Job drawing, mm, ordinate dimensions from the low corner. One solid piece. Round coordinates to 2 decimals unless told otherwise and drop trailing zeros. Order: outer loops, then holes, each group sorted by start corner. A loop starts at its lowest first (then second) coordinate and runs counter-clockwise, first axis right, second up. Notation, with made-up numbers: (-21, 87.25) -> (27, 87.25) arc R30 ccw to (27, 113.25) -> close; hole circle Ø9 at (59.25, 17.5). An arc over 180 degrees is marked (long way). Answer as a JSON object with one key per item and string values. Group by question number.
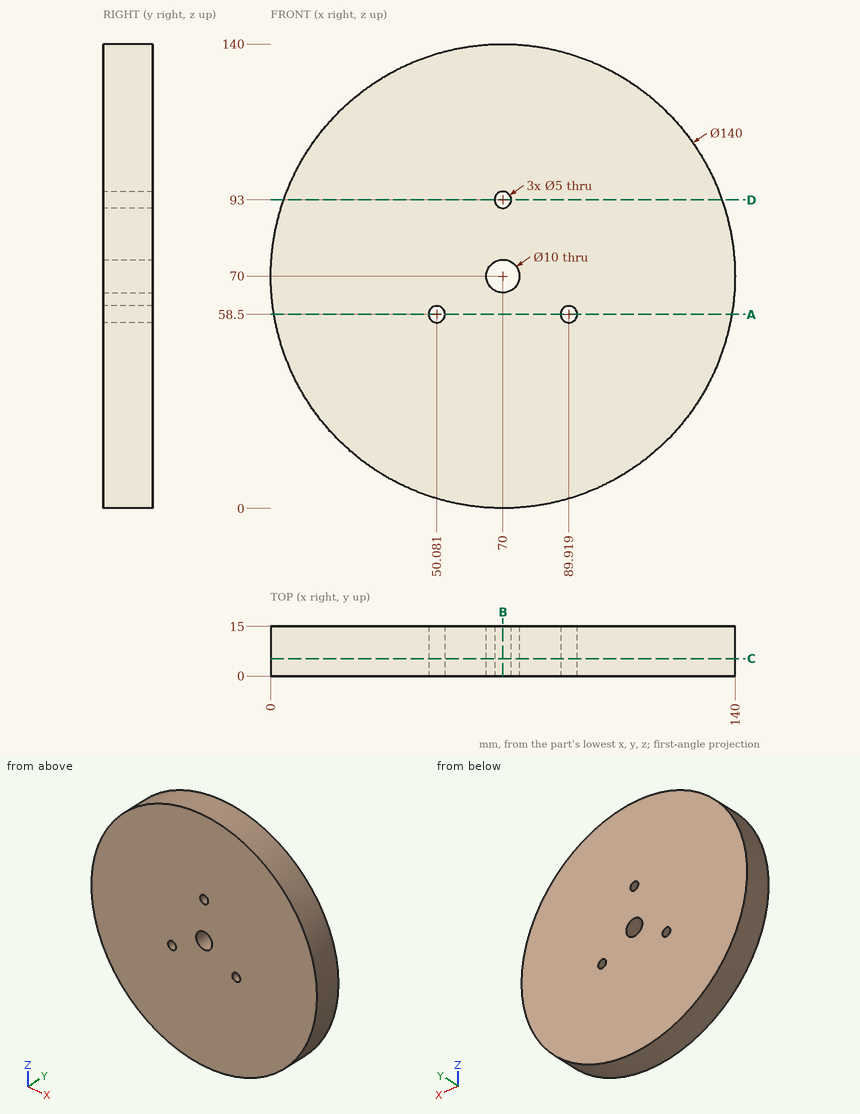
Q1. Band-saw the part on B-B (x = 70). List the corners of the cut face in (y, z), plus the area to 4 significant figures.
Q2. Band-saw the part on A-A (z = 58.5). List the corners of the cut face in (x, y), plus the area to 3 significant figures.
Q3. Band-saw the part on D-D (z = 93). List the corners of the cut face in (x, y), plus the area to 3 significant figures.
Q4. Band-saw the part on C-C (y = 5.25). List the corners of the cut face in (x, z).
Q5. Drop flat-ended pins along their axis: pin 1 Ø6 at (y, z) = (8.5, 33) entering from +X; pin 2 Ø4 at (y, z) = (9, 62) entering from +X; pin 3 Ø4 at (x, y) = (103.5, 1.5) entering from -Z. Give the stop position or say it passes through.
Q6. Wall check: line 1 (Z direction, x = 70, y = 7.75); line 2 (X direction, y = 8, z = 58); line 3 (X direction, y = 4.25, z = 70). Give the ranges that are in metal, low to high. Write a range as [from, to].
Completed:
{
 "1": {"outline": "(0, 0) -> (15, 0) -> (15, 65) -> (0, 65) -> close; (0, 75) -> (15, 75) -> (15, 90.5) -> (0, 90.5) -> close; (0, 95.5) -> (15, 95.5) -> (15, 140) -> (0, 140) -> close", "area": "1,875 mm2"},
 "2": {"outline": "(0.95, 0) -> (47.58, 0) -> (47.58, 15) -> (0.95, 15) -> close; (52.58, 0) -> (87.42, 0) -> (87.42, 15) -> (52.58, 15) -> close; (92.42, 0) -> (139.05, 0) -> (139.05, 15) -> (92.42, 15) -> close", "area": "1,920 mm2"},
 "3": {"outline": "(3.89, 0) -> (67.5, 0) -> (67.5, 15) -> (3.89, 15) -> close; (72.5, 0) -> (136.11, 0) -> (136.11, 15) -> (72.5, 15) -> close", "area": "1,910 mm2"},
 "4": {"outline": "circle Ø140 at (70, 70); hole circle Ø5 at (50.08, 58.5); hole circle Ø10 at (70, 70); hole circle Ø5 at (70, 93); hole circle Ø5 at (89.92, 58.5)"},
 "5": {"pin 1": "x = 131.19", "pin 2": "x = 139.74", "pin 3": "z = 7.49"},
 "6": {"line 1": "[0, 65], [75, 90.5], [95.5, 140]", "line 2": "[1.04, 47.63], [52.53, 87.47], [92.37, 138.96]", "line 3": "[0, 65], [75, 140]"}
}
